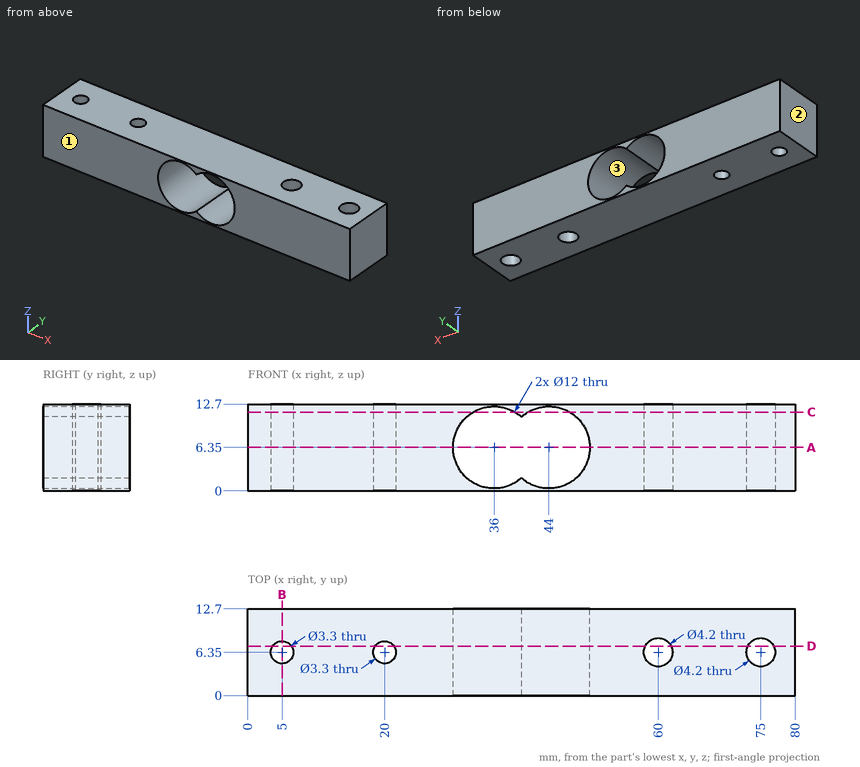
Input: dimensioned drawing with shaded views. Units: mm. Origin: part minimum x, y, z. Coordinates: 2 decimals unless noted, no trailing zeros. Order: outer loops, then holes, each group sorted by start corner. A loop starts at its lowest first (then second) coordinate and runs counter-clockwise, first axis right, second up. Notation, with made-up numbers: (81, -18) - (99, -18) arc R13 ccw to (99, 3) - close; hole circle Ø6 at (31, 78.5). An arc over 180 degrees is marked (long way). Return JSON: item names as keys, results as strings. Group by question number.
1. Cut plane A-A (z = 6.35). Output: boundary loops of the cut face in (x, y).
2. Pin query (flat end, axial travel): pin 1 (1.5 mm diameter, centred on y = 7, z = 6, fed in from -X). Return the tip coordinate at first contact, or that it passes through.
3. Pull-direction query (X, two-part tool) for the marked faces 1, 2 and 3; classes: pulls with the +X half, pulls with the -X half, needs draft (parallel to the pull), parting line crosses it, or undercut.
4. Cut plane C-C (z = 11.5). Output: boundary loops of the cut face in (x, y), plus the area to 3 significant figures.
5. Cut plane D-D (y = 7.25). Output: boundary loops of the cut face in (x, z).
6. Cut plane B-B (x = 5). Output: boundary loops of the cut face in (y, z).
7. Material intervals for line 1 along Z through (x, y) = (44, 7); line 2 along Y through (x, z) = (20, 3); line 3 along X through (y, z) = (7, 4), sorted ascending. Write a range as [from, to].
Resolved:
{
 "1": {"outline": "(0, 0) - (30, 0) - (30, 12.7) - (0, 12.7) - close; (50, 0) - (80, 0) - (80, 12.7) - (50, 12.7) - close; hole circle Ø3.3 at (5, 6.35); hole circle Ø3.3 at (20, 6.35); hole circle Ø4.2 at (60, 6.35); hole circle Ø4.2 at (75, 6.35)"},
 "2": {"pin 1": "stops at x = 0"},
 "3": {"face 1": "needs draft", "face 2": "pulls with the -X half", "face 3": "undercut"},
 "4": {"outline": "(0, 0) - (32.92, 0) - (32.92, 12.7) - (0, 12.7) - close; (39.08, 0) - (40.92, 0) - (40.92, 12.7) - (39.08, 12.7) - close; (47.08, 0) - (80, 0) - (80, 12.7) - (47.08, 12.7) - close; hole circle Ø3.3 at (5, 6.35); hole circle Ø3.3 at (20, 6.35); hole circle Ø4.2 at (60, 6.35); hole circle Ø4.2 at (75, 6.35)", "area": "815 mm²"},
 "5": {"outline": "(0, 0) - (3.62, 0) - (3.62, 12.7) - (0, 12.7) - close; (6.38, 0) - (18.62, 0) - (18.62, 12.7) - (6.38, 12.7) - close; (21.38, 0) - (58.1, 0) - (58.1, 12.7) - (21.38, 12.7) - close; (61.9, 0) - (73.1, 0) - (73.1, 12.7) - (61.9, 12.7) - close; (76.9, 0) - (80, 0) - (80, 12.7) - (76.9, 12.7) - close; hole (40, 1.88) arc R6 ccw (long way) to (40, 10.82) arc R6 ccw (long way) to start"},
 "6": {"outline": "(0, 0) - (4.7, 0) - (4.7, 12.7) - (0, 12.7) - close; (8, 0) - (12.7, 0) - (12.7, 12.7) - (8, 12.7) - close"},
 "7": {"line 1": "z = [0, 0.35], [12.35, 12.7]", "line 2": "y = [0, 4.7], [8, 12.7]", "line 3": "x = [0, 3.48], [6.52, 18.48], [21.52, 30.48], [49.52, 58], [62, 73], [77, 80]"}
}
